Study the drawing (mm; zero at the part's minimum x, y, z) and answer. A direction names the side the tool comes from. Give positions to 0.01 mm unless a question says otherwise; leave off trailing zeros. Order: outer loops, then holes, each group sorted by start corner. A loop starts at its lowest first (then second) coordinate and runs counter-clockwise, first axis right, second up. Notation, with made-up numbers: (47.5, -33.5) -> (56.5, -33.5) arc R22 cw to (56.5, -25.5) -> close; hole circle Ø1 at (86.5, 69.5). An arc over 180 degrees is marked (long way). Use a Markdown table: item, result. Add a question column.
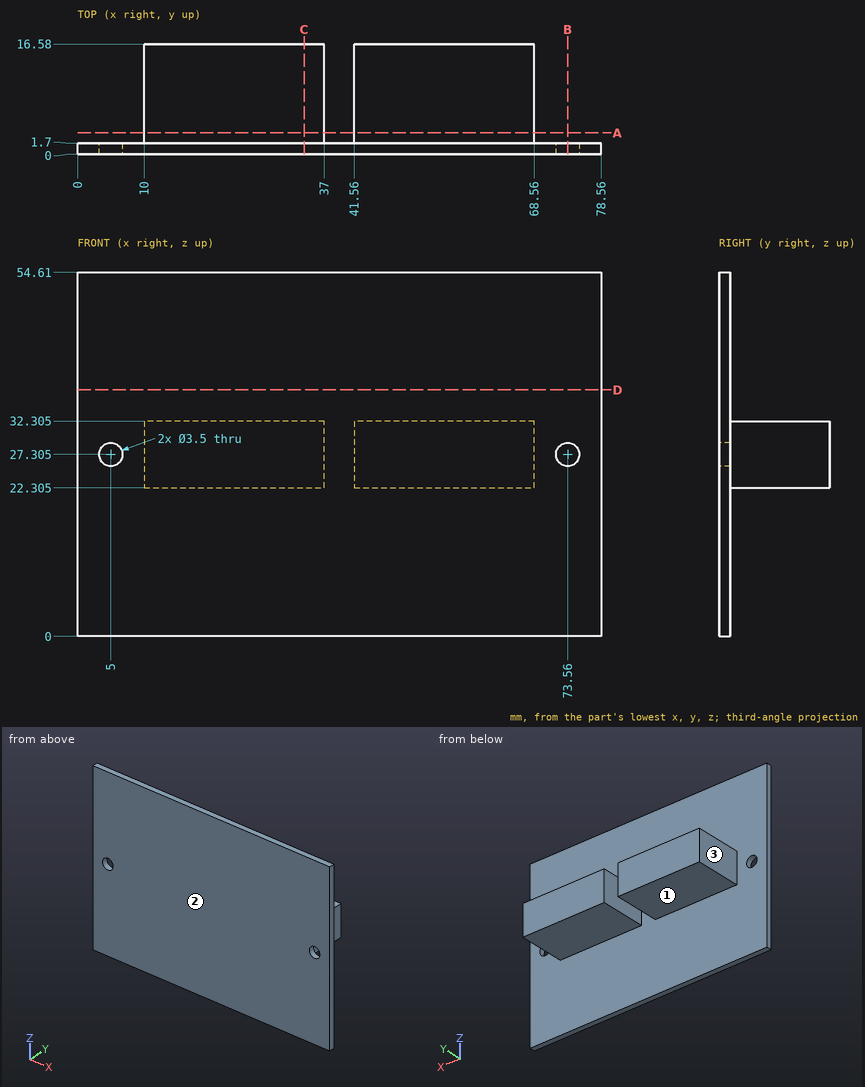
1) Flat-ended cylindrical pins translate along their axes: pin 1 (5 mm diameter, centred on y = 7.5, z = 29.5, fed in from -X); pin 2 (1 mm diameter, centred on x = 64, y = 14, fed in from +Z) (3 decimals); pin 3 (8 mm diameter, centred on y = 8, z = 29, fed in from +X). Find the tip coordinate at first contact, or state that the pin passes through.
2) The part is cut by section B-B, the plane x = 73.56. Determine the outline of the cut face in (y, z) (3 decimals).
3) The part is cut by section C-C, the plane x = 34. Determine the outline of the cut face in (y, z) (3 decimals).
4) Straight lines are drawn through the part: line 1 (Z direction, x = 5, y = 1.25) (3 decimals); line 2 (X direction, y = 10.75, z = 25); line 3 (Z direction, x = 42, y = 8.25) (3 decimals). For each, find the intervals that lie inside material, in ascending order.
5) The part is cut by section A-A, the plane y = 3.25. Determine the outline of the cut face in (x, z) (3 decimals), then the cut area to 3 significant figures.
6) The part is cut by section D-D, the plane z = 37. Determine the outline of the cut face in (x, y), then the cut area to 3 significant figures.
7) Which of the six approach directions +Z, -Z, +X, -X, +Y, -Y give full straight-line access (tool end or side, diameter ignored) to the marked faces 1, 2 and 3?
A:
| question | item | result |
|---|---|---|
| 1 | pin 1 | x = 10 |
| 1 | pin 2 | z = 32.305 |
| 1 | pin 3 | x = 68.56 |
| 2 | outline | (0, 0) -> (1.7, 0) -> (1.7, 25.555) -> (0, 25.555) -> close; (0, 29.055) -> (1.7, 29.055) -> (1.7, 54.61) -> (0, 54.61) -> close |
| 3 | outline | (0, 0) -> (1.7, 0) -> (1.7, 22.305) -> (16.58, 22.305) -> (16.58, 32.305) -> (1.7, 32.305) -> (1.7, 54.61) -> (0, 54.61) -> close |
| 4 | line 1 | 0 to 25.555, 29.055 to 54.61 |
| 4 | line 2 | 10 to 37, 41.56 to 68.56 |
| 4 | line 3 | 22.305 to 32.305 |
| 5 | outline | (10, 22.305) -> (37, 22.305) -> (37, 32.305) -> (10, 32.305) -> close; (41.56, 22.305) -> (68.56, 22.305) -> (68.56, 32.305) -> (41.56, 32.305) -> close |
| 5 | area | 540 mm^2 |
| 6 | outline | (0, 0) -> (78.56, 0) -> (78.56, 1.7) -> (0, 1.7) -> close |
| 6 | area | 134 mm^2 |
| 7 | face 1 | -Z, +X, -X, +Y |
| 7 | face 2 | +Z, -Z, +X, -X, -Y |
| 7 | face 3 | +Z, -Z, -X, +Y |
